Source: CAD feature listing. Evaluate the final solid. Frame: model axes, mm. Face numbers are marked on the shaded views. A direction names the side the tool comes from. Give positions to 0.01 mm unless a question says otherwise; leave off trailing zeros. Loops run counter-clockwise (first coordinate to the right, second up) from the corner with the lowest first, then second, coordinate; pieces in that order, holes last. Notation, with made-up numbers: (-37.75, -28.75) -> (-31.75, -28.75) arc R17 cw to (-31.75, -2.75) -> close; hole circle Ø1 at (1.5, 30.5). An arc over 180 degrees is marked (long way). Put each result on its own line as item: value.
```python
from build123d import *

# Parameters (mm, degrees)
F0_R      = 14
F0_R_2    = 10.25
F1_DEPTH  = 70
F4_DEPTH  = 40
F5_SIZE   = 3
F6_D      = 3.3
F7_R      = 0.2
F10_DEPTH = 40


with BuildPart() as f1:
    # F0 (on Front) → F1 (new body)
    with BuildSketch(Plane.XZ):
        Circle(F0_R)
        Circle(F0_R_2, mode=Mode.SUBTRACT)
    extrude(amount=F1_DEPTH)

    # F3 (on offset) → F4 (cut)
    with BuildSketch(Plane.YZ.offset(14)):
        with BuildLine():
            Line((-70.0558224349, -6.4983871577), (-47.1447907046, -6.4983871577))
            ThreePointArc((-47.1447907046, -6.4983871577), (-40.5004032231, -0.0723998436), (-47, 6.5))
            Line((-47, 6.5), (-70.0558218767, 6.5))
            Line((-70.0558218767, 6.5), (-70.0558224349, -6.4983871577))
        make_face()
    extrude(amount=-F4_DEPTH, mode=Mode.SUBTRACT)

    # F5
    f5_edges = [f1.edges().sort_by_distance(p)[0] for p in [
        (0, -70, 10.25),
        (0, -70, -10.25),
    ]]
    chamfer(f5_edges, length=F5_SIZE)

    # F6 (through all)
    with Locations(Plane.YZ.offset(14)):
        with Locations((-5, 0)):
            Hole(F6_D / 2)

    # F7
    f7_edges = [f1.edges().sort_by_distance(p)[0] for p in [
        (-14, 0, 0),
    ]]
    fillet(f7_edges, radius=F7_R)

    # F9 (on offset) → F10 (cut)
    with BuildSketch(Plane.XY.offset(14)):
        with BuildLine():
            Line((6.5, -70.223480463), (6.5, -47))
            ThreePointArc((6.5, -47), (0, -40.5), (-6.5, -47))
            Line((-6.5, -47), (-6.5, -70.1674371958))
            Line((-6.5, -70.1674371958), (6.5, -70.223480463))
        make_face()
    extrude(amount=-F10_DEPTH, mode=Mode.SUBTRACT)


solid = f1.part
```
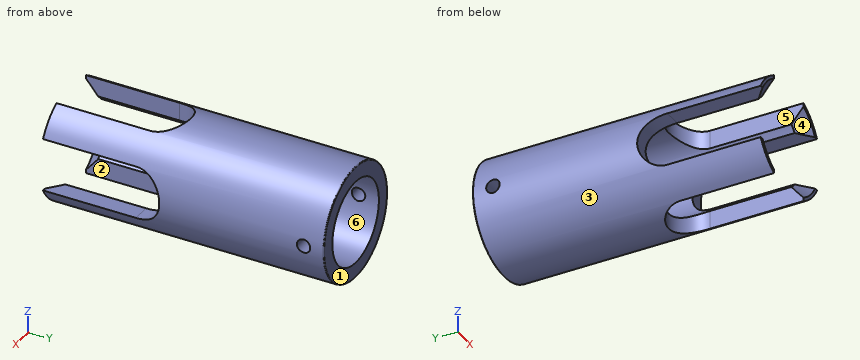
(1) Section B-B on x = 0. Return loops of the section in (y, z).
Calculated:
outline: (-40.5, -14) -> (-0.2, -14) arc R0.2 ccw to (0, -13.8) -> (0, -10.25) -> (-40.5, -10.25) -> close; (-40.5, 10.25) -> (0, 10.25) -> (0, 13.8) arc R0.2 ccw to (-0.2, 14) -> (-40.5, 14) -> close
(2) First-contact query: P1, Ø3.5, axis at x = 10.5, y = -57, coming from the -Z side; P2, Ø4, axis at x = -10.5, y = -36.5, coming from the +Z side; P3, Ø3.5, axis at x = -11, y = -56, coming from the +Z side. Flat tips, straight axial feed; report the tip coordinate or a pass-through.
Calculated:
P1: stops at z = -10.93
P2: stops at z = 11.12
P3: stops at z = 10.51
(3) Section D-D on y = -5. Return loops of the section in (x, z), then the cut area to 3 significant figures.
Calculated:
outline: (-13.9, -1.65) arc R14 ccw to (13.9, -1.65) -> (10.12, -1.65) arc R10.25 cw to (-10.12, -1.65) -> close; (-13.9, 1.65) -> (-10.12, 1.65) arc R10.25 cw to (10.12, 1.65) -> (13.9, 1.65) arc R14 ccw to start
area: 261 mm²
(4) Section C-C on z = 0. Return loops of the section in (x, y).
Calculated:
outline: (-14, -40.5) -> (-10.25, -40.5) -> (-10.25, -6.65) -> (-14, -6.65) -> close; (-14, -3.35) -> (-10.25, -3.35) -> (-10.25, 0) -> (-13.8, 0) arc R0.2 ccw to (-14, -0.2) -> close; (10.25, -40.5) -> (14, -40.5) -> (14, -6.65) -> (10.25, -6.65) -> close; (10.25, -3.35) -> (14, -3.35) -> (14, -0.2) arc R0.2 ccw to (13.8, 0) -> (10.25, 0) -> close
(5) Line query: probe 1 along Z at (x, y) = (0, -34.5); probe 2 along Z at (x, y) = (6.5, -4). Output: solid intervals per line, ascending. Write a range as from..to.
Calculated:
probe 1: z = -14..-10.25, 10.25..14
probe 2: z = -12.4..-7.93, 7.93..12.4
(6) Section A-A on y = -55. Return loops of the section in (x, z), then the cut area to 3 significant figures.
Calculated:
outline: (-12.4, -6.5) arc R14 ccw to (-6.5, -12.4) -> (-6.5, -7.93) arc R10.25 cw to (-7.93, -6.5) -> close; (-12.4, 6.5) -> (-7.93, 6.5) arc R10.25 cw to (-6.5, 7.93) -> (-6.5, 12.4) arc R14 ccw to start; (6.5, -12.4) arc R14 ccw to (12.4, -6.5) -> (7.93, -6.5) arc R10.25 cw to (6.5, -7.93) -> close; (6.5, 7.93) arc R10.25 cw to (7.93, 6.5) -> (12.4, 6.5) arc R14 ccw to (6.5, 12.4) -> close
area: 79.5 mm²
(7) Draft query along X for the marked faces 1, 2, 3 and 4. Return one class per face: released by +X, released by -X, zero draft, split by the parting line, or undercut.
Calculated:
face 1: zero draft
face 2: undercut
face 3: split by the parting line
face 4: undercut
(8) Reachability of the marked faces 5 and 6 from +Z, -Z, +X, -X, +Y, -Y: full face, straight path, thin tool, end or side. Return the list, or none.
Calculated:
face 5: +Z, -Z, -Y
face 6: +Y, -Y
